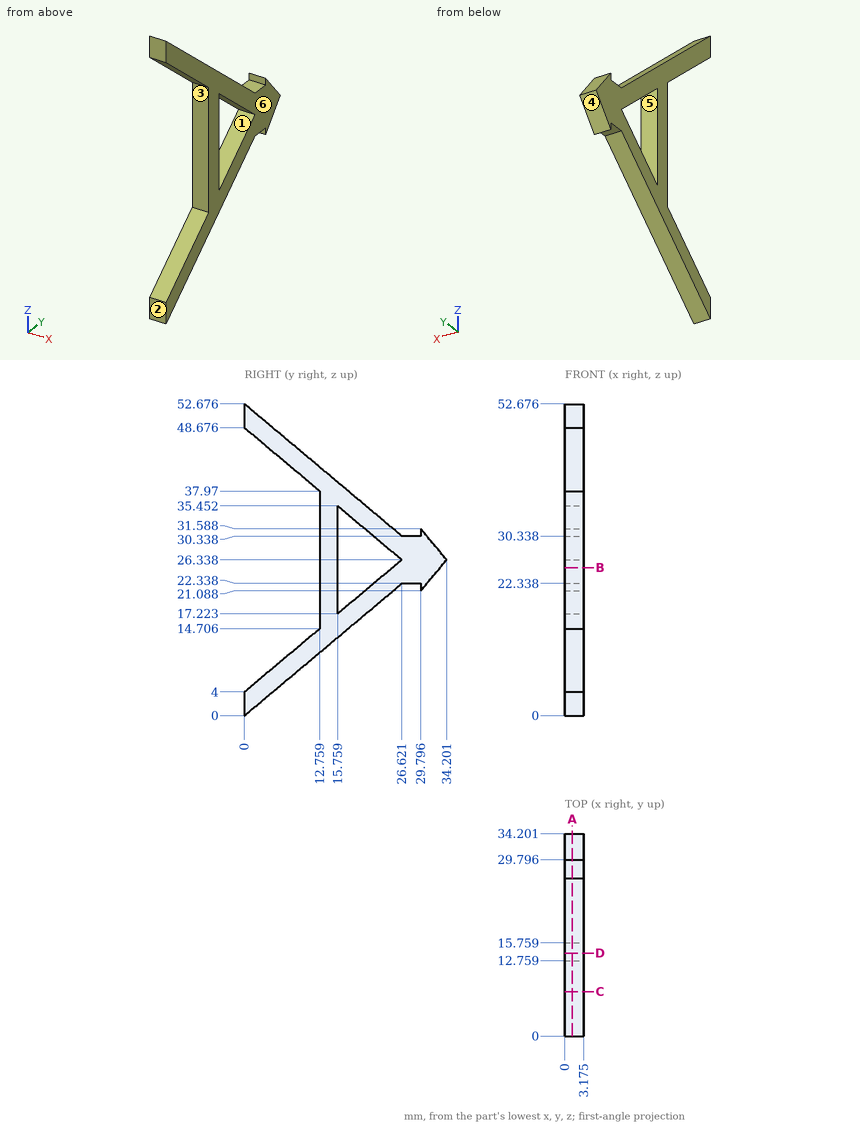
Design review of the part shown in the three views and the two pictorial views. Dimensions are in mm from the part's minimum x, y and z. A direction names the side the tool comes from. Coordinates: 2 decimals unless noted, no trailing zeros. Order: outer loops, then holes, each group sorted by start corner. A loop starts at its lowest first (then second) coordinate and runs counter-clockwise, first axis right, second up.
Item 1: For pin 1 Ø1.4 at (x, z) = (2, 22) entering from -Y, flat-tipped, find the tip position at first contact; note if it passes through.
Item 2: Take a section at D-D, the plane y = 14. Write out the cut boundary in (x, z) (1 decimal).
Item 3: The part is to be moulded in two halves that separate along Y. For the marked faces 4, 5 and 6, say which applies: pulls with the +Y half, pulls with the -Y half, needs draft (parallel to the pull), parting line crosses it, or undercut.
Item 4: For line 1 (Z direction, x = 1.2, y = 5.5) (1 decimal); line 2 (Z direction, x = 1.5, y = 3.5) (1 decimal); line 3 (Y direction, x = 0.9, z = 38.5) (1 decimal), list the stretches that pass through material, from the lowest coordinate up.
Item 5: For the marked faces 1, 2 and 3, list the 3-axis set-ups (+Z, -Z, +X, -X, +Y, -Y) from which the entire face can be reached by the end or side of a thin tool; tool diameter is ignored.
Item 6: Take a section at A-A, the plane x = 1.3. Write out the cut boundary in (y, z) (1 decimal).
Item 7: Take a section at B-B, the plane z = 25. Write out the cut boundary in (x, y) (1 decimal).
Item 8: Take a section at C-C, the plane y = 7.5. Write out the cut boundary in (x, z) (1 decimal), then the cut area to 3 significant figures.
The answers:
1. pin 1: stops at y = 12.76
2. outline: (0, 11.7) - (3.2, 11.7) - (3.2, 40.9) - (0, 40.9) - close
3. face 4: pulls with the +Y half
3. face 5: undercut
3. face 6: needs draft
4. line 1: z = 4.6 to 8.6, 44.1 to 48.1
4. line 2: z = 2.9 to 6.9, 45.7 to 49.7
4. line 3: y = 12.1 to 16.9
5. face 1: +X, -X
5. face 2: +Z, -Z, +X, -X, -Y
5. face 3: +X, -X, -Y
6. outline: (0, 0) - (26.6, 22.3) - (29.8, 22.3) - (29.8, 21.1) - (34.2, 26.3) - (29.8, 31.6) - (29.8, 30.3) - (26.6, 30.3) - (0, 52.7) - (0, 48.7) - (12.8, 38) - (12.8, 14.7) - (0, 4) - close; hole (15.8, 17.2) - (26.6, 26.3) - (15.8, 35.5) - close
7. outline: (0, 12.8) - (3.2, 12.8) - (3.2, 15.8) - (0, 15.8) - close; (0, 25) - (3.2, 25) - (3.2, 33.1) - (0, 33.1) - close
8. outline: (0, 6.3) - (3.2, 6.3) - (3.2, 10.3) - (0, 10.3) - close; (0, 42.4) - (3.2, 42.4) - (3.2, 46.4) - (0, 46.4) - close
8. area: 25.4 mm2
